Design review of the part shown in the three views and the two pictorial views. Dimensions are in mm from the part's minimum x, y and z. A direction names the side the tool comes from. Coordinates: 2 decimals unless noted, no trailing zeros. Loops run counter-clockwise (first coordinate to the right, second up) from the corner with the lowest first, then second, coordinate; pieces in that order, holes last. Notation, with made-up numbers: (64.5, -36.75) -> (96.5, -36.75) arc R25 ccw to (96.5, 1.25) -> close; hole circle Ø7 at (42.25, 32.25). An arc over 180 degrees is marked (long way). Answer in a Markdown table with one row per item.
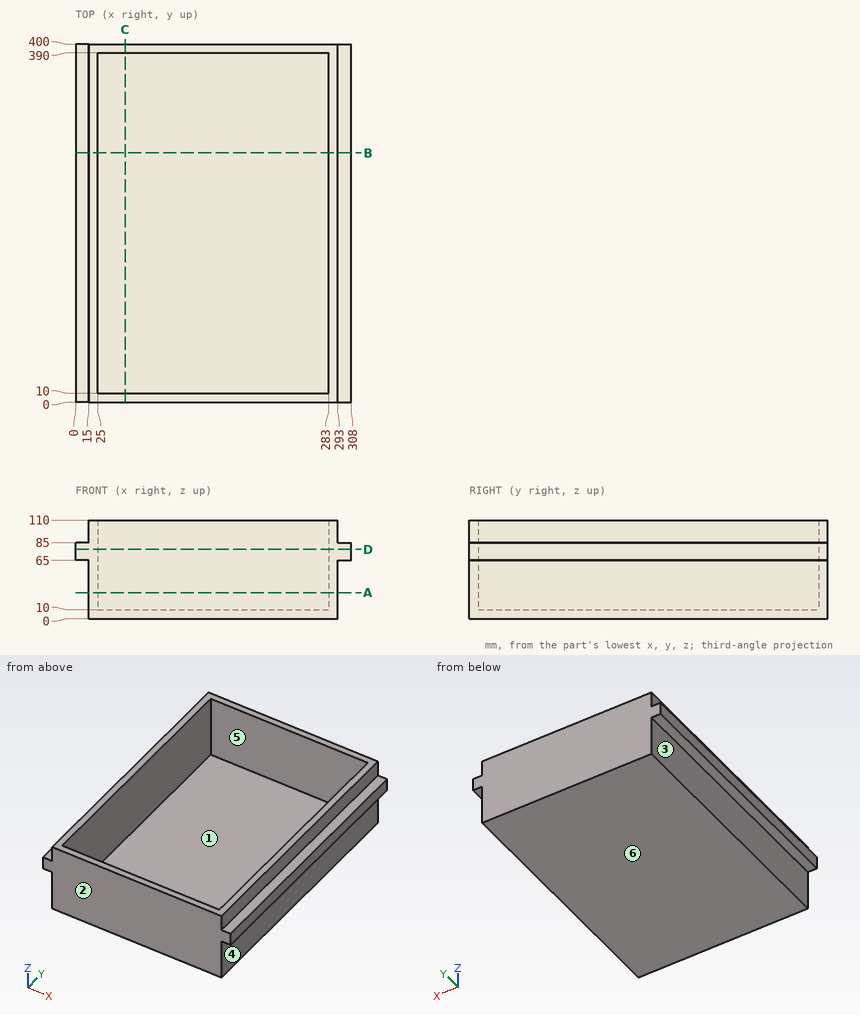
Item 1: For L1, parallel to Y at x = 256.5, z = 46; L2, parallel to X at y = 237, z = 92; L3, parallel to X at y = 276.5, z = 77, list the stretches that pass through material, from the lowest coordinate up.
Worked answers:
| item | result |
|---|---|
| L1 | 0 to 10, 390 to 400 |
| L2 | 15 to 25, 283 to 293 |
| L3 | 0 to 25, 283 to 308 |
Item 2: Take a section at D-D, the plane z = 77.5. State the section outline as (x, y) points.
Worked answers:
| item | result |
|---|---|
| outline | (0, 0) -> (308, 0) -> (308, 400) -> (0, 400) -> close; hole (25, 10) -> (283, 10) -> (283, 390) -> (25, 390) -> close |
Item 3: For the marked faces 4, 5 and 6, list the 3-axis set-ups (+Z, -Z, +X, -X, +Y, -Y) from which the entire face can be reached by the end or side of a thin tool; tool diameter is ignored.
Worked answers:
| item | result |
|---|---|
| face 4 | -Z, +X, +Y, -Y |
| face 5 | +Z |
| face 6 | -Z, +X, -X, +Y, -Y |
Item 4: Take a section at C-C, the plane x = 55.5. State the section outline as (y, z) points.
Worked answers:
| item | result |
|---|---|
| outline | (0, 0) -> (400, 0) -> (400, 110) -> (390, 110) -> (390, 10) -> (10, 10) -> (10, 110) -> (0, 110) -> close |
Item 5: The part is to be moulded in two halves that separate along Y. For the marked faces 1, 2 and 3, say which applies: +Y half, -Y half, draft (parallel to the pull), parting line (faces both ways), or undercut.
Worked answers:
| item | result |
|---|---|
| face 1 | undercut |
| face 2 | -Y half |
| face 3 | draft |
Item 6: Take a section at A-A, the plane z = 29. State the section outline as (x, y) points.
Worked answers:
| item | result |
|---|---|
| outline | (15, 0) -> (293, 0) -> (293, 400) -> (15, 400) -> close; hole (25, 10) -> (283, 10) -> (283, 390) -> (25, 390) -> close |
Item 7: Take a section at B-B, the plane y = 278.5. State the section outline as (x, z) points.
Worked answers:
| item | result |
|---|---|
| outline | (0, 65) -> (15, 65) -> (15, 0) -> (293, 0) -> (293, 65) -> (308, 65) -> (308, 85) -> (293, 85) -> (293, 110) -> (283, 110) -> (283, 10) -> (25, 10) -> (25, 110) -> (15, 110) -> (15, 85) -> (0, 85) -> close |
Item 8: Insertion check: pin 1 (2 mm diameter, centred on y = 195, z = 37.5, fed in from +X); pin 2 (4.5 mm diameter, centred on x = 301.5, y = 299.5, fed in from +Z); pin 3 (5 mm diameter, centred on x = 157.5, y = 108.5, fed in from -Z); pin 4 (10 mm diameter, centred on x = 228, y = 247, fed in from +Z). Each pin has a flat end and moves straight along its axis. Give the tip position at first contact, or say it passes through.
Worked answers:
| item | result |
|---|---|
| pin 1 | x = 293 |
| pin 2 | z = 85 |
| pin 3 | z = 0 |
| pin 4 | z = 10 |
